Read the model definition and answer for the solid it produces. Units are mm, in the model's axes. A direction names the side the tool comes from. Round coordinates to 2 decimals unless told otherwise and drop trailing zeros. Loops run counter-clockwise (first coordinate to the right, second up) from the corner with the lowest first, then second, coordinate; pieces in that order, holes last. Notation, with made-up numbers: M -21.5,62.5 L 12.5,62.5 A23 cw 12.5,74.5 Z; hole C 23.5,74 d10. An arc over 180 degrees is marked long. Write each question's results on one line, items separated by ' | '.
```python
from build123d import *

# Parameters (mm, degrees)
SKETCH1_R           = 8
BOSS_EXTRUDE1_DEPTH = 22
SKETCH2_R           = 5.1
CUT_EXTRUDE1_DEPTH  = 13
SKETCH4_R           = 9.9
BOSS_EXTRUDE2_DEPTH = 1.5
CUT_EXTRUDE2_DEPTH  = 23


with BuildPart() as part:
    # Sketch1 → Boss-Extrude1 (new body)
    with BuildSketch(Plane.XY):
        Circle(SKETCH1_R)
    extrude(amount=BOSS_EXTRUDE1_DEPTH)

    # Sketch2 → Cut-Extrude1 (cut)
    with BuildSketch(Plane.XY.offset(22)):
        Circle(SKETCH2_R)
    extrude(amount=-CUT_EXTRUDE1_DEPTH, mode=Mode.SUBTRACT)

    # Sketch4 → Boss-Extrude2 (add)
    with BuildSketch(Plane(origin=(0, 0, 0), x_dir=(-1, 0, 0), z_dir=(0, 0, -1))):
        Circle(SKETCH4_R)
    extrude(amount=-BOSS_EXTRUDE2_DEPTH)

    # Sketch3 → Cut-Extrude2 (cut, through all)
    with BuildSketch(Plane(origin=(0, 0, 0), x_dir=(-1, 0, 0), z_dir=(0, 0, -1))):
        with BuildLine():
            Line((-0.858778202, 1.35), (0.858778202, 1.35))
            ThreePointArc((0.858778202, 1.35), (0, -1.6), (-0.858778202, 1.35))
        make_face()
    extrude(amount=-CUT_EXTRUDE2_DEPTH, mode=Mode.SUBTRACT)


solid = part.part
```
1. Determine the mould class of faces 3 (the face through (-9.443, 2.974, 0.74)), 4 (the face through (0, 1.35, 4)), 5 (the face through (2, 0, 9)), 6 (the face through (3.7, -7.3, 1.5)) for opening direction Y: released by +Y, released by -Y, zero draft, split by the parting line, or undercut.
Completed:
face 3: split by the parting line | face 4: undercut | face 5: undercut | face 6: zero draft
2. Which of the six approach directions +Z, -Z, +X, -X, +Y, -Y give full straight-line access (tool end or side, diameter ignored) to faces 1 (the face through (0, -2, 0)), 2 (the face through (-1.73, -7.81, 11.61))?
Completed:
face 1: -Z, +X, -X, +Y, -Y | face 2: +Z
3. Find section A-A, the plane y = 0. Give the vertices of the cut face in (x, z).
Completed:
outline: M -9.9,0 L -1.6,0 L -1.6,9 L -5.1,9 L -5.1,22 L -8,22 L -8,1.5 L -9.9,1.5 Z; M 1.6,0 L 9.9,0 L 9.9,1.5 L 8,1.5 L 8,22 L 5.1,22 L 5.1,9 L 1.6,9 Z
4. Find the intervals of material crossed by L1, parallel to Y at x = 0, z = 14.5; L2, parallel to Y at x = 0, z = 6.5; L3, parallel to X at y = 0, z = 2.25, in increasing order.
Completed:
L1: y = -8 to -5.1, 5.1 to 8 | L2: y = -8 to -1.6, 1.35 to 8 | L3: x = -8 to -1.6, 1.6 to 8
5. Given P1, Ø2, axis at y = 8, z = 12, coming from the -X side; P2, Ø0.9, axis at x = 0.5, z = 5.5, coming from the -Y side; P3, Ø1.5, axis at y = -1.5, z = 10, coming from the +X side; P4, Ø6, axis at x = 2, y = -4, coming from the +Z side, each flat-ended and moving along its own axis, determine where each tip first touches the part or whether it passes through.
Completed:
P1: stops at x = -3.87 | P2: stops at y = -8 | P3: stops at x = 7.96 | P4: stops at z = 22
6. Find section C-C, the plane z = 18. Give the vertices of the cut face in (x, y), then the cut area to 3 significant figures.
Completed:
outline: C 0,0 d16; hole C 0,0 d10.2 | area: 119 mm2
7. Find section D-D, the plane x = 6. Give the vertices of the cut face in (y, z), then the cut area to 3 significant figures.
Completed:
outline: M -7.87,0 L 7.87,0 L 7.87,1.5 L 5.29,1.5 L 5.29,22 L -5.29,22 L -5.29,1.5 L -7.87,1.5 Z | area: 241 mm2
8. Find section B-B, the plane x = 0. Give the vertices of the cut face in (y, z).
Completed:
outline: M -9.9,0 L -1.6,0 L -1.6,9 L -5.1,9 L -5.1,22 L -8,22 L -8,1.5 L -9.9,1.5 Z; M 1.35,0 L 9.9,0 L 9.9,1.5 L 8,1.5 L 8,22 L 5.1,22 L 5.1,9 L 1.35,9 Z
